from build123d import *

# Parameters (mm, degrees)
BOSS_EXTRUDE1_DEPTH = 25
SKETCH3_R           = 2
CUT_EXTRUDE1_DEPTH  = 15
SKETCH2_W           = 4
SKETCH2_H           = 26
BOSS_EXTRUDE2_DEPTH = 20
SKETCH7_W           = 15
SKETCH7_H           = 5
BOSS_EXTRUDE4_DEPTH = 25
CUT_EXTRUDE2_DEPTH  = 20
BOSS_EXTRUDE5_DEPTH = 4
CUT_EXTRUDE3_START  = -10
SKETCH10_R          = 2
CUT_EXTRUDE3_DEPTH  = 10
SKETCH11_W          = 15
SKETCH11_H          = 15
BOSS_EXTRUDE6_DEPTH = 14
SKETCH14_W          = 15
SKETCH14_H          = 15
CUT_EXTRUDE5_DEPTH  = 0.5
BOSS_EXTRUDE7_DEPTH = 5
SKETCH13_R          = 2
CUT_EXTRUDE6_DEPTH  = 10
SKETCH17_W          = 20
SKETCH17_H          = 11.5
CUT_EXTRUDE7_DEPTH  = 1


with BuildPart() as part:
    # Sketch1 → Boss-Extrude1 (new body)
    with BuildSketch(Plane.XY):
        Polygon((15.200344072, 13.760447293), (0.200344072, 13.760447293), (0.200344072, -6.239552707), (-4.799655928, -6.239552707), (-4.799655928, 19.760447293), (15.200344072, 19.760447293), align=None)
    extrude(amount=BOSS_EXTRUDE1_DEPTH)

    # Sketch3 → Cut-Extrude1 (cut)
    with BuildSketch(Plane.XZ.offset(-13.760447293)):
        with Locations((7.700344072, 21.5)):
            Circle(SKETCH3_R)
    extrude(amount=-CUT_EXTRUDE1_DEPTH, mode=Mode.SUBTRACT)

    # Sketch2 → Boss-Extrude2 (add)
    with BuildSketch(Plane.ZY.offset(4.799655928)):
        with Locations((2, 6.760447293)):
            Rectangle(SKETCH2_W, SKETCH2_H)
    extrude(amount=-BOSS_EXTRUDE2_DEPTH)

    # Sketch7 → Boss-Extrude4 (add)
    with BuildSketch(Plane.XY.offset(4)):
        with Locations((7.700344072, -3.739552707)):
            Rectangle(SKETCH7_W, SKETCH7_H)
    extrude(amount=BOSS_EXTRUDE4_DEPTH)

    # Sketch8 → Cut-Extrude2 (cut)
    with BuildSketch(Plane(origin=(15.200344072, 0, 0), x_dir=(0, 0, -1), z_dir=(1, 0, 0))):
        Polygon((-4, -1.239552707), (-4, -6.239552707), (0, -6.239552707), (0, 19.760447293), (-4, 19.760447293), (-4, 13.760447293), align=None)
    extrude(amount=-CUT_EXTRUDE2_DEPTH, mode=Mode.SUBTRACT)

    # Sketch9 → Boss-Extrude5 (add)
    with BuildSketch(Plane.XY.offset(25)):
        Polygon((15.200344072, 13.760447293), (15.200344072, 19.760447293), (-4.799655928, 19.760447293), (-4.799655928, -6.239552707), (0.200344072, -6.239552707), (0.200344072, -1.239552707), (0.200344072, 13.760447293), align=None)
    extrude(amount=BOSS_EXTRUDE5_DEPTH)

    # Sketch10 → Cut-Extrude3 (cut)
    with BuildSketch(Plane(origin=(0, -1.239552707, 0), x_dir=(1, 0, 0), z_dir=(0, 1, 0)).offset(CUT_EXTRUDE3_START)):
        with Locations((7.700344072, -21.5)):
            Circle(SKETCH10_R)
    extrude(amount=CUT_EXTRUDE3_DEPTH, mode=Mode.SUBTRACT)

    # Sketch11 → Boss-Extrude6 (add)
    with BuildSketch(Plane(origin=(0, 0, 4), x_dir=(-1, 0, 0), z_dir=(0, 0, -1))):
        with Locations((-7.700344072, 6.260447293)):
            Rectangle(SKETCH11_W, SKETCH11_H)
    extrude(amount=-BOSS_EXTRUDE6_DEPTH)

    # Sketch14 → Cut-Extrude5 (cut)
    with BuildSketch(Plane.XY.offset(18)):
        with Locations((7.700344072, 6.260447293)):
            Rectangle(SKETCH14_W, SKETCH14_H)
    extrude(amount=-CUT_EXTRUDE5_DEPTH, mode=Mode.SUBTRACT)

    # Sketch16 → Boss-Extrude7 (add)
    with BuildSketch(Plane(origin=(15.200344072, 0, 0), x_dir=(0, 0, -1), z_dir=(1, 0, 0))):
        Polygon((-29, 13.760447293), (-17.5, 13.760447293), (-17.5, -1.239552707), (-29, -1.239552707), (-29, -6.239552707), (-4, -6.239552707), (-4, 19.760447293), (-29, 19.760447293), align=None)
    extrude(amount=BOSS_EXTRUDE7_DEPTH)

    # Sketch13 → Cut-Extrude6 (cut)
    with BuildSketch(Plane(origin=(0, 0, 4), x_dir=(-1, 0, 0), z_dir=(0, 0, -1))):
        with Locations(Location((-14.700344072, -0.239552707, 0), (0, 0, 90))):
            Circle(SKETCH13_R)
        with Locations(Location((-14.700344072, 13.760447293, 0), (0, 0, 90))):
            Circle(SKETCH13_R)
        with Locations(Location((-0.700344072, 13.760447293, 0), (0, 0, 90))):
            Circle(SKETCH13_R)
        with Locations(Location((-0.700344072, -0.239552707, 0), (0, 0, 90))):
            Circle(SKETCH13_R)
    extrude(amount=-CUT_EXTRUDE6_DEPTH, mode=Mode.SUBTRACT)

    # Sketch17 → Cut-Extrude7 (cut)
    with BuildSketch(Plane.XZ.offset(-13.760447293)):
        with Locations((10.200344072, 23.25)):
            Rectangle(SKETCH17_W, SKETCH17_H)
    extrude(amount=-CUT_EXTRUDE7_DEPTH, mode=Mode.SUBTRACT)


solid = part.part
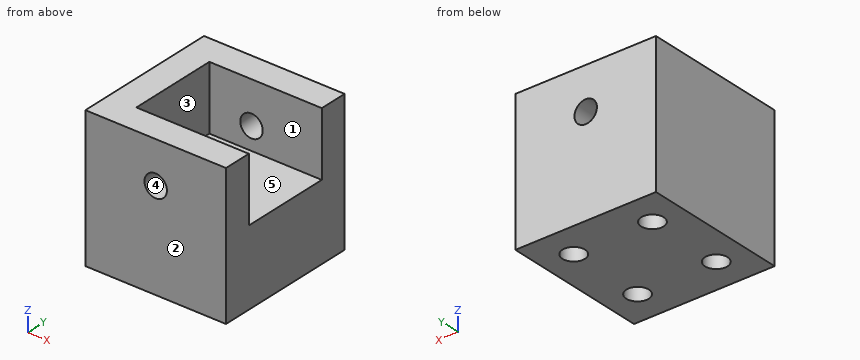
Source: CAD feature listing. Evaluate the final solid. Frame: model axes, mm. Face numbers are marked on the shaded views. A direction names the side the tool comes from. Round coordinates to 2 decimals unless told otherwise and drop trailing zeros. Loops run counter-clockwise (first coordinate to the right, second up) from the corner with the lowest first, then second, coordinate; pieces in that order, holes last.
Q1. Ray query, line 1 (Y direction, x = 16.5, z = 24.25); line 2 (Y direction, x = 14.75, z = 12.75); line 3 (X direction, y = 1.5, z = 8.5). Return the intervals inside material, ascending.
Q2. Section A-A, the plane z = 21.5. Return loops of the section in (x, y), plus the area to 3 significant figures.
Q3. First-contact query: P1, Ø2, axis at x = 1.5, y = -0.5, coming from the -Z side; P2, Ø6, axis at y = 5, z = 25, coming from the +X side. Flat tips, straight axial feed; report the tip coordinate or a pass-through.
Q4. Section C-C, the plane y = 7. Return loops of the section in (x, z).
Q5. Section B-B, the plane x = 6.75. Return loops of the section in (y, z).
Q6. Access query for the marked faces 1 and 2. Directions: +Z, -Z, +X, -X, +Y, -Y. A direction counts if a zero-diameter tool reaches every point of the face in a straight line with its end or side. Return the directions, or none.
Q7. Section D-D, the plane y = 17.25. Return loops of the section in (x, z), plus the area to 3 significant figures.
Q8. Mould query, pull axis Z, two halves, no side actions, for the marked faces 3, 4 and 5. Classes: pulls with the +Z half, pulls with the -Z half, needs draft (parallel to the pull), parting line crosses it, or undercut.
Solutions:
1. line 1: y = -6.24 to -1.24, 14.76 to 19.76
1. line 2: y = -6.24 to -2.24, 1.76 to 11.76, 15.76 to 19.76
1. line 3: x = -4.8 to -0.29, 1.69 to 13.71, 15.69 to 20.2
2. outline: (-4.8, -6.24) - (5.7, -6.24) - (5.7, -1.24) - (0.2, -1.24) - (0.2, 14.76) - (5.7, 14.76) - (5.7, 19.76) - (-4.8, 19.76) - close; (9.7, -6.24) - (20.2, -6.24) - (20.2, -1.24) - (9.7, -1.24) - close; (9.7, 14.76) - (20.2, 14.76) - (20.2, 19.76) - (9.7, 19.76) - close
2. area: 290 mm2
3. P1: stops at z = 14
3. P2: stops at x = 0.2
4. outline: (-4.8, 4) - (20.2, 4) - (20.2, 17.5) - (0.2, 17.5) - (0.2, 29) - (-4.8, 29) - close
5. outline: (-6.24, 4) - (19.76, 4) - (19.76, 19.74) - (14.76, 19.74) - (14.76, 17.5) - (-1.24, 17.5) - (-1.24, 19.74) - (-6.24, 19.74) - close; (-6.24, 23.26) - (-1.24, 23.26) - (-1.24, 29) - (-6.24, 29) - close; (14.76, 23.26) - (19.76, 23.26) - (19.76, 29) - (14.76, 29) - close
6. face 1: +Z, +X
6. face 2: +Z, -Z, +X, -X, -Y
7. outline: (-4.8, 4) - (20.2, 4) - (20.2, 29) - (-4.8, 29) - close; hole circle Ø4 at (7.7, 21.5)
7. area: 612 mm2
8. face 3: needs draft
8. face 4: undercut
8. face 5: pulls with the +Z half
